Autodesk Inventor part; units mm, degrees
ref_plane "YZ Plane" through (0, 0, 0) normal (1, 0, 0) x (0, 1, 0)
ref_plane "XZ Plane" through (0, 0, 0) normal (0, 1, 0) x (-1, 0, 0)
ref_plane "XY Plane" through (0, 0, 0) normal (0, 0, 1) x (1, 0, 0)
sketch "スケッチ1" plane through (0, 0, 0) normal (0, 0, 1) x (1, 0, 0)
  circle A0 centre (-15.5, 0) radius 2.5
  circle A1 centre (15.5, 0) radius 2.5
  circle A2 centre (0, 0) radius 11
  line L0 (-15.1987, 13) -> (15.1987, 13)
  arc A3 (15.1987, -13) -> (15.1987, 13) centre (0, 0) ccw
  line L1 (15.1987, -13) -> (-15.1987, -13)
  arc A4 (-15.1987, 13) -> (-15.1987, -13) centre (0, 0) ccw
  circle A5 centre (-15.5, -130.182) radius 2.5
  circle A6 centre (15.5, -130.182) radius 2.5
  circle A7 centre (0, -130.182) radius 11
  line L2 (-15.1987, -143.182) -> (15.1987, -143.182)
  arc A8 (-15.1987, -117.182) -> (-15.1987, -143.182) centre (0, -130.182) ccw
  line L3 (15.1987, -117.182) -> (-15.1987, -117.182)
  arc A9 (15.1987, -143.182) -> (15.1987, -117.182) centre (0, -130.182) ccw
  circle A10 centre (0, -130.182) radius 5
  circle A11 centre (0, 0) radius 5
  line L4 (-29, -33.3404) -> (-29, 14.9098)
  line L5 (99, -145.0893) -> (-29, -145.0893)
  line L6 (-29, -63.34) -> (-29, -33.3408)
  line L7 (99, -145.0893) -> (99, 14.9098)
  line L8 (99, 14.9098) -> (297.1795, 14.9098)
  line L9 (297.1795, 14.9098) -> (297.1795, -145.0893)
  line L10 (297.1795, -145.0893) -> (99, -145.0893)
  circle A12 centre (0, -130.1819) radius 55
  circle A13 centre (0, 0.0009) radius 55
  line L11 (297.1795, -145.0893) -> (237.1795, -145.0893)
  line L12 (237.1795, -145.0893) -> (237.1795, 14.9098)
  line L13 (237.1795, 14.9098) -> (297.1795, 14.9098)
  line L14 (297.1795, 14.9098) -> (297.1795, -145.0893)
  line L15 (99, 14.9098) -> (-29, 14.9098)
  line L16 (99, 14.9098) -> (99, -145.0893)
  line L17 (92, -168.0902) -> (92, 36.9098)
  line L18 (86, 36.9098) -> (86, -168.0902)
  line L19 (89, 7.9098) -> (89, -7.0902) construction
  line L20 (92, 7.9098) -> (92, -7.0902)
  line L21 (86, -7.0902) -> (86, 7.9098)
  arc A14 (92, 7.9098) -> (86, 7.9098) centre (89, 7.9098) ccw
  arc A15 (86, -7.0902) -> (92, -7.0902) centre (89, -7.0902) ccw
  line L22 (87.3545, -74.7724) -> (87.3545, -54.7724) construction
  line L23 (90.3545, -74.7724) -> (90.3545, -54.7724)
  line L24 (84.3545, -54.7724) -> (84.3545, -74.7724)
  arc A16 (84.3545, -74.7724) -> (90.3545, -74.7724) centre (87.3545, -74.7724) ccw
  arc A17 (90.3545, -54.7724) -> (84.3545, -54.7724) centre (87.3545, -54.7724) ccw
  line L25 (-29, -145.0893) -> (-0.25, -145.0893)
  line L26 (-0.25, -145.0893) -> (-0.25, 14.9098)
  line L27 (-0.25, 14.9098) -> (-29, 14.9098)
  line L28 (-29, 14.9098) -> (-29, -145.0893)
  line L29 (19.75, -105.0893) -> (19.75, -25.0893)
  line L30 (19.75, -25.0893) -> (-20.25, -25.0893)
  line L31 (-20.25, -25.0893) -> (-20.25, -105.0893)
  line L32 (-20.25, -105.0893) -> (19.75, -105.0893)
  line L33 (19.75, -105.0893) -> (-20.25, -25.0893) construction
  line L34 (19.75, -25.0893) -> (-20.25, -105.0893) construction
  line L35 (19.75, -110.0893) -> (19.75, -20.0893)
  line L36 (19.75, -20.0893) -> (-20.25, -20.0893)
  line L37 (-20.25, -20.0893) -> (-20.25, -110.0893)
  line L38 (-20.25, -110.0893) -> (19.75, -110.0893)
  line L39 (19.75, -110.0893) -> (-20.25, -20.0893) construction
  line L40 (19.75, -20.0893) -> (-20.25, -110.0893) construction
  circle A18 centre (19.75, -110.0893) radius 1.5
  circle A19 centre (19.75, -20.0893) radius 1.5
  circle A20 centre (-20.25, -20.0893) radius 1.5
  circle A21 centre (-20.25, -110.0893) radius 1.5
  line L41 (88.9576, -138.0893) -> (88.9576, -123.0893) construction
  line L42 (91.9576, -138.0893) -> (91.9576, -123.0893)
  line L43 (85.9576, -123.0893) -> (85.9576, -138.0893)
  arc A22 (85.9576, -138.0893) -> (91.9576, -138.0893) centre (88.9576, -138.0893) ccw
  arc A23 (91.9576, -123.0893) -> (85.9576, -123.0893) centre (88.9576, -123.0893) ccw
  line L44 (-15.829, -33.3462) -> (-29, -33.3404)
  line L45 (-29, -145.0893) -> (-29, -63.34)
  line L46 (-29, -63.34) -> (-16.162, -63.34)
  arc A24 (-16.162, -63.34) -> (-15.829, -33.3462) centre (-16.25, -48.3403) ccw
  line L47 (55.6416, -41.2467) -> (55.6416, -91.2467)
  arc A25 (55.6416, -91.2467) -> (80.6416, -91.2467) centre (68.1416, -91.2467) ccw
  line L48 (80.6416, -91.2467) -> (80.6416, -41.2467)
  arc A26 (80.6416, -41.2467) -> (55.6416, -41.2467) centre (68.1416, -41.2467) ccw
  line L49 (86, -55.0898) -> (86, -75.0898)
  arc A27 (86, -75.0898) -> (92, -75.0898) centre (89, -75.0898) ccw
  line L50 (92, -75.0898) -> (92, -55.0898)
  arc A28 (92, -55.0898) -> (86, -55.0898) centre (89, -55.0898) ccw
  circle A29 centre (48.7299, -140.0893) radius 1.5
  circle A30 centre (14.75, -81.84) radius 15.8
  circle A31 centre (-15.5, 0.0016) radius 2.5
  circle A32 centre (-15.5, -130.1804) radius 2.5
  arc A33 (86.1416, -121.2458) -> (90.1416, -121.2458) centre (88.1416, -121.2458) ccw
  line L51 (90.1416, -121.2458) -> (90.1416, -111.2458)
  arc A34 (90.1416, -111.2458) -> (86.1416, -111.2458) centre (88.1416, -111.2458) ccw
  line L52 (86.1416, -111.2458) -> (86.1416, -121.2458)
  arc A35 (56.1416, -21.2467) -> (60.1416, -21.2467) centre (58.1416, -21.2467) ccw
  line L53 (60.1416, -21.2467) -> (60.1416, -11.2467)
  arc A36 (60.1416, -11.2467) -> (56.1416, -11.2467) centre (58.1416, -11.2467) ccw
  line L54 (56.1416, -11.2467) -> (56.1416, -21.2467)
  arc A37 (92, 9.9098) -> (86, 9.9098) centre (89, 9.9098) ccw
  line L55 (86, 9.9098) -> (86, -0.0902)
  arc A38 (86, -0.0902) -> (92, -0.0902) centre (89, -0.0902) ccw
  line L56 (92, -0.0902) -> (92, 9.9098)
  arc A39 (56.1416, -121.2458) -> (60.1416, -121.2458) centre (58.1416, -121.2458) ccw
  line L57 (60.1416, -121.2458) -> (60.1416, -111.2458)
  arc A40 (60.1416, -111.2458) -> (56.1416, -111.2458) centre (58.1416, -111.2458) ccw
  line L58 (56.1416, -111.2458) -> (56.1416, -121.2458)
  circle A41 centre (68.7415, -140.0893) radius 1.5
  circle A42 centre (0, -130.1803) radius 6.7
  circle A43 centre (15.5, 0.0016) radius 2.5
  circle A44 centre (0, 0.0017) radius 6.7
  circle A45 centre (15.5, -130.1804) radius 2.5
  circle A46 centre (48.73, 9.9098) radius 1.5
  arc A47 (86, -140.0893) -> (92, -140.0893) centre (89, -140.0893) ccw
  line L59 (92, -140.0893) -> (92, -130.0893)
  arc A48 (92, -130.0893) -> (86, -130.0893) centre (89, -130.0893) ccw
  line L60 (86, -130.0893) -> (86, -140.0893)
  arc A49 (90.1416, -11.2467) -> (86.1416, -11.2467) centre (88.1416, -11.2467) ccw
  line L61 (86.1416, -11.2467) -> (86.1416, -21.2467)
  arc A50 (86.1416, -21.2467) -> (90.1416, -21.2467) centre (88.1416, -21.2467) ccw
  line L62 (90.1416, -21.2467) -> (90.1416, -11.2467)
  line L63 (40.1416, -63.2467) -> (36.1416, -63.2467)
  arc A51 (36.1416, -63.2467) -> (36.1416, -69.2467) centre (36.1416, -66.2467) ccw
  line L64 (36.1416, -69.2467) -> (40.1416, -69.2467)
  arc A52 (40.1416, -69.2467) -> (40.1416, -63.2467) centre (40.1416, -66.2467) ccw
  circle A53 centre (68.9885, 9.909) radius 1.5
  circle A54 centre (68.9885, 9.9098) radius 1.5
  line L65 (99, -145.0893) -> (79, -145.0893)
  line L66 (79, -145.0893) -> (79, 14.9098)
  line L67 (79, 14.9098) -> (99, 14.9098)
  line L68 (99, 14.9098) -> (99, -145.0893)
  point P0 (0, 0)
  point P1 (119, 14.909)
  point P2 (89, 0.4098)
  point P3 (92, 7.909)
  point P4 (92, -7.091)
  point P5 (86, -7.094)
  point P6 (86, 7.9142)
  point P7 (87.3545, -64.7724)
  point P8 (86, -7.0941)
  point P9 (86, 7.909)
  point P10 (92, -55.0901)
  point P11 (92, -75.0901)
  point P12 (86, -77.4492)
  point P13 (86, -52.0956)
  point P14 (114.2151, 14.909)
  point P15 (237.2519, 14.9098)
  point P16 (-0.25, -65.0893)
  point P17 (86, -7.0943)
  point P18 (86, -7.091)
  point P19 (88.9576, -130.5893)
  point P20 (86, -138.5921)
  point P21 (86, -122.5866)
  point P22 (112.6121, 14.909)
  point P23 (112.6121, 14.909)
  point P24 (92.6121, -145.0901)
  point P25 (92.6121, 14.909)
  point P26 (-0.25, -145.0901)
  point P27 (92.6121, 14.909)
  point P28 (-0.25, -145.0901)
  point P29 (237.1795, -145.0893)
  point P30 (237.1795, 14.909)
  point P31 (-29, -33.3412)
  point P32 (-29, -63.3408)
  point P33 (-0.25, -145.091)
  point P34 (-29, -33.3422)
  point P35 (-29, -63.3417)
  point P36 (-0.25, -145.091)
  point P37 (-0.25, -145.0908)
  point P38 (-0.25, -145.0908)
  point P39 (-0.25, -145.0905)
  point P40 (-0.25, -145.0905)
  point P41 (-0.25, -145.0902)
  point P42 (-0.25, -145.0902)
  point P43 (-0.25, -145.0899)
  point P44 (-0.25, -145.0899)
  point P45 (-0.25, -145.0896)
  point P46 (-0.25, -145.0896)
  point P47 (-0.25, -145.0893)
  point P48 (-0.25, -145.0893)
  point P49 (-13, -0.0021)
  point P50 (-18, 0.0038)
  point P51 (18, -0.0021)
  point P52 (13, 0.0038)
  point P53 (86, -7.0943)
  point P54 (-13, -130.1782)
  point P55 (-18, -130.1841)
  point P56 (18, -130.1782)
  point P57 (13, -130.1841)
  point P58 (92, -55.0881)
  point P59 (92, -75.0915)
  point P60 (86, -75.0915)
  point P61 (86, -55.0881)
  dimension "d2" = 110
  dimension "d3" = 110
  dimension "d4" = 60
  dimension "d5" = 159.9991
  dimension "d10" = 7
  dimension "d11" = 15
  dimension "d12" = 6
  dimension "d14" = 20
  dimension "d17" = 80
  dimension "d18" = 40
  dimension "d19" = 159.9991
  dimension "d20" = 80
  dimension "d21" = 90
  dimension "d22" = 40
  dimension "d23" = 3
  dimension "d24" = 3
  dimension "d25" = 3
  dimension "d26" = 3
  dimension "d27" = 15
  dimension "d29" = 7
  dimension "d30" = 20
extrude "押し出し1" add sketch "スケッチ1" along normal blind 1 contours A2 L26 A44 | A2 L26 L0 A3 L1 | L26 A44 A2 | A2 L26 L1 A4 L0 | L26 L15 A13 L29 L35 A19 L36 L1 A3 L0 | L0 A4 L1 L26 L36 A20 L37 L31 L44 L4 L15 | L36 A19 L35 L30 L26 | L26 L30 L37 A20 L36 | L15 L66 A26 L47 A25 L5 A12 A30 L29 A13 | L30 L29 A13 L26 | L26 A13 A24 L44 L31 L30 | L44 L31 A13 L6 | A13 L31 L46 L6 | L15 L18 A17 L24 A16 A23 L43 A22 L5 L66 A25 L48 A26 | L26 A12 L31 L46 A24 A13 | A13 L29 A30 A12 L26 | L44 A24 A13 L31 | L46 L31 A12 L28 | A13 A24 L46 L31 | L15 L17 A37 L18 | L66 A25 L47 A26 | A26 L48 A25 L66 | L26 A30 L32 L31 A12 | A12 A30 L26 | A30 A12 L29 | L29 A12 A30 | A12 L31 L37 A21 L38 L26 L3 A8 L2 L5 L28 | L15 L7 L5 L17 | A37 L17 A14 L18 | A12 L29 A30 L26 | L26 A30 | A12 A30 L29 | L5 L26 L2 A9 L3 L38 A18 L35 L29 A30 A12 | L32 L26 L38 A21 L37 | A30 L29 L32 L26 | L18 A47 L17 L5 | L32 L35 A18 L38 L26 | L26 A7 L3 A9 L2 | L2 A8 L3 L26 A7 | A15 A49 L61 A50 L62 L17 A28 A17 L18 | L18 A22 L42 A48 L17 A47 | L26 A42 A7 | A7 L26 A42 | A17 A28 L18 | L18 A16 L24 A17 | A15 A49 L62 A50 L61 | A22 L43 A23 L18 | A48 L42 A23 L51 A34 L52 A33 L18 A16 A27 L17 | A27 A16 L18 | A33 L52 A34 L51 A23 | A29 | L54 A36 L53 A35 | L58 A40 L57 A39 | A41 | A46 | A53
sketch "スケッチ2" plane through (0, 0, 0) normal (0, 0, -1) x (-1, 0, 0)
  point P0 (0, 0)
fillet "フィレット1" radius 5 4 edges at (-29, -145.0893, 0.5) (-29, 14.9098, 0.5) (99, -145.0893, 0.5) (99, 14.9098, 0.5)
properties part number "前方後方板"
Design review of the part built by this model. Coordinates are the model's own, in mm. Coordinates: 2 decimals unless noted, no trailing zeros. Order: outer loops, then holes, each group sorted by start corner. A loop starts at its lowest first (then second) coordinate and runs counter-clockwise, first axis right, second up.
1) Mouldability with a two-part tool opening along Y and no side actions: class faces 1 (the cylindrical face through (13, -0.1, 0.5)), 2 (the cylindrical face through (97.5, -143.66, 0.51)), 3 (the cylindrical face through (-27.5, 13.48, 0.51)) as +Y half, -Y half, draft (parallel to the pull), parting line (faces both ways), or undercut.
2) Take a section at C-C, the plane x = 15.5. Give the boundary of the cut face in (y, z), and give its area (3 significant figures).
3) Clearance check with flat-ended pins moving along their axes: pin 1 (21.5 mm diameter, centred on x = 0, y = -130.18, fed in from -Z); pin 2 (1.8 mm diameter, centred on x = 19.75, y = -20.09, fed in from +Z). State where each tip first meets the part, or that it passes through.
4) Wall thickness on line 1 along Y through (x, z) = (0, 0.4); line 2 along Y through (x, z) = (-15.5, 0.75); line 3 along X through (y, z) = (-59.5, 0.2): over which ranges is each line inside the solid? List them lowest first.
5) Take a section at D-D, the plane z = 0.5. State how many separate pieces and enclosed holes the cut face has, and give its area (3 significant figures).
6) Take a section at A-A, the plane x = 0. Give the boundary of the cut face in (y, z), and give its area (3 significant figures).
7) Take a section at B-B, the plane x = 89. Give the boundary of the cut face in (y, z).
Returned:
1. face 1: undercut
1. face 2: -Y half
1. face 3: +Y half
2. outline: (-145.09, 0) - (-132.68, 0) - (-132.68, 1) - (-145.09, 1) - close; (-127.68, 0) - (-2.5, 0) - (-2.5, 1) - (-127.68, 1) - close; (2.5, 0) - (14.91, 0) - (14.91, 1) - (2.5, 1) - close
2. area: 150 mm2
3. pin 1: stops at z = 0
3. pin 2: passes through
4. line 1: y = -145.09 to -136.88, -123.48 to -6.7, 6.7 to 14.91
4. line 2: y = -145.09 to -132.68, -127.68 to -2.5, 2.5 to 14.91
4. line 3: x = -29 to 86, 92 to 99
5. separate pieces: 1
5. enclosed holes: 14
5. area: 19,600 mm2
6. outline: (-145.09, 0) - (-136.88, 0) - (-136.88, 1) - (-145.09, 1) - close; (-123.48, 0) - (-6.7, 0) - (-6.7, 1) - (-123.48, 1) - close; (6.7, 0) - (14.91, 0) - (14.91, 1) - (6.7, 1) - close
6. area: 133 mm2
7. outline: (-145.09, 0) - (-141.09, 0) - (-141.09, 1) - (-145.09, 1) - close; (-120.09, 0) - (-78.09, 0) - (-78.09, 1) - (-120.09, 1) - close; (-52.09, 0) - (-10.09, 0) - (-10.09, 1) - (-52.09, 1) - close; (10.91, 0) - (14.91, 0) - (14.91, 1) - (10.91, 1) - close
